Check sheet for the modelled part. Datum: model origin and axes. Units: mm. A direction names the side the tool comes from. Give positions to 0.01 mm unless a question says otherwise; leave off trailing zeros. Write each loop counter-clockwise with the first axis right and the second up, starting at its lowest first coordinate (ties: lowest second). Pieces come first, ordered by that corner, then holes. Notation, with made-up numbers: M -24,-34.75 L 25,-34.75 A32 cw 25,-4.75 Z; hole C 10,79.25 d11. An arc over 180 degrees is marked long. Use CSV: the item, a comma, the result in double quotes. Start each with the question number.
1. Cross-section at B-B, the plane y = 2. Enter the section's corners in (x, z).
2. Depth check by flat-ended pin: P1, Ø6, axis at x = 11, z = -0.5, coming from the -Y side; P2, Ø3, axis at y = 0, z = -2, coming from the +X side; P3, Ø1, axis at y = 4, z = -2.5, coming from the +X side; P4, Ø3, axis at x = 14.5, y = 6, coming from the +Z side. Enter the tip coordinate at first touch or a pass-through.
3. Access from +Z, -Z, +X, -X, +Y, -Y to the whole of each face (thin tool, end or side, straight path). Record for faces 1 (the face through (11, 5, 0)), 2 (the face through (1, 0, 5)).
4. Cross-section at A-A, the plane x = 3.5. Enter the section's corners in (y, z), and give its area (3 significant figures).
5. Cross-section at C-C, the plane z = -2.25. Enter the section's corners in (x, y), and give its area (3 significant figures).
6. Scan lines: line 1 (Z direction, x = -12, y = -6); line 2 (X direction, y = 6, z = 2); line 3 (X direction, y = -3, z = -7.5). Record each from-to range of solid material in increasing order.
from build123d import *

# Parameters (mm, degrees)
F1_DEPTH = 5
F2_R     = 11.905945
F3_DEPTH = 15


with BuildPart() as f1:
    # F0 (on Top) → F1 (new body)
    with BuildSketch(Plane.XY):
        Polygon((17.539468, 0), (5.419994, 16.681025), (-14.189727, 10.30944), (-14.189727, -10.30944), (5.419994, -16.681025), align=None)
    extrude(amount=F1_DEPTH)

    # F2 (on face) → F3 (join)
    with BuildSketch(Plane.XY.offset(5)):
        Circle(F2_R)
    extrude(amount=-F3_DEPTH)


solid = f1.part
Worked answers:
1,outline,"M -14.19,0 L -11.74,0 L -11.74,-10 L 11.74,-10 L 11.74,0 L 16.09,0 L 16.09,5 L -14.19,5 Z"
2,P1,"stops at y = -13.07"
2,P2,"stops at x = 11.91"
2,P3,"stops at x = 11.38"
2,P4,"stops at z = 5"
3,face 1,"-Z"
3,face 2,"+Z, +X, -X, +Y, -Y"
4,outline,"M -16.06,0 L -11.38,0 L -11.38,-10 L 11.38,-10 L 11.38,0 L 16.06,0 L 16.06,5 L -16.06,5 Z"
4,area,"388 mm^2"
5,outline,"C 0,0 d23.81"
5,area,"445 mm^2"
6,line 1,"z = 0 to 5"
6,line 2,"x = -14.19 to 13.18"
6,line 3,"x = -11.52 to 11.52"
